Answer from the drawing. Dimensions are ordinates in mm from the lowest x, y and z of the part. A direction names the side the tool comes from. Give positions to 0.01 mm unless a question says otherwise; leave off trailing zeros. Write each loop counter-clockwise with the first axis right and the second up, starting at its lowest first coordinate (ties: lowest second). Pieces come first, ordered by that corner, then holes. Notation, with made-up numbers: (28.5, 76) -> (39.5, 76) arc R17 cw to (39.5, 99) -> close; hole circle Ø8 at (36.5, 1). An arc over 180 degrees is marked (long way). Write item = value, one per line.
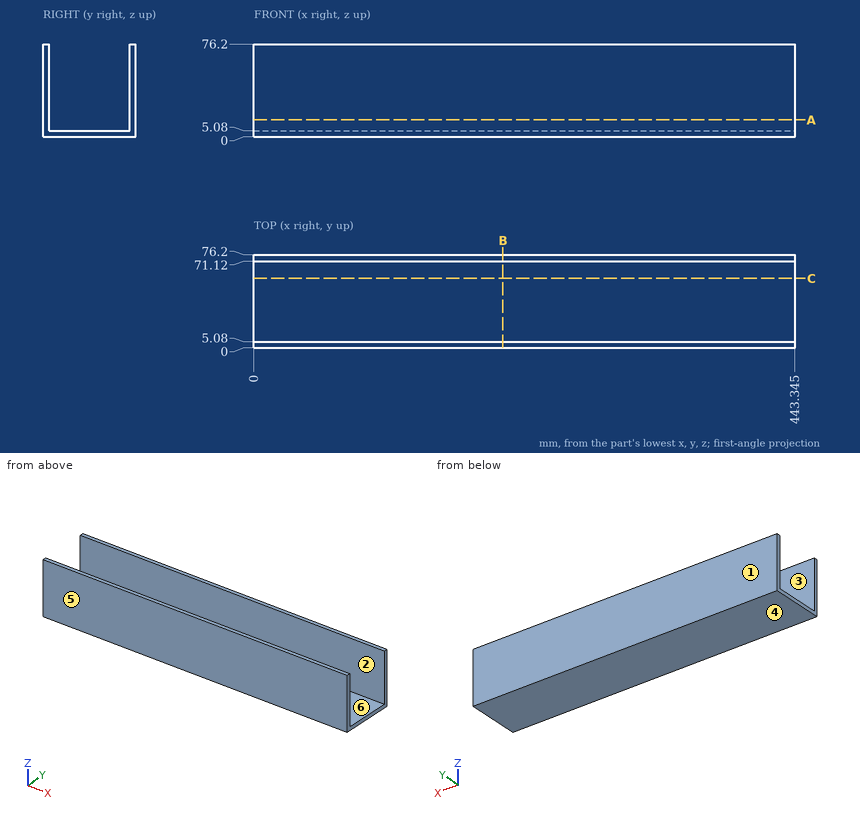
(1) For a pull along Y with two mould halves and no side action, classify the marked faces 3, 4, 5 and 6 as released by +Y, released by -Y, zero draft, split by the parting line, or undercut.
Checks:
face_3 = undercut
face_4 = zero draft
face_5 = released by -Y
face_6 = undercut
(2) Given P1, Ø5, axis at x = 126.5, y = 13, coming from the +Z side; P2, Ø8, axis at x = 189.5, y = 59, coming from the -Z side, each flat-ended and moving along its own axis, determine where each tip first touches the part or whether it passes through.
Checks:
P1 = 5.08
P2 = 0
(3) The part is cut by section B-B on x = 204. Determine the outline of the cut face in (y, z).
Checks:
outline = (0, 0) -> (76.2, 0) -> (76.2, 76.2) -> (71.12, 76.2) -> (71.12, 5.08) -> (5.08, 5.08) -> (5.08, 76.2) -> (0, 76.2) -> close
(4) A tool of negligible diameter and unlimited length cuts with its end or side. For the marked faces 1 and 2, from which of +Z, -Z, +X, -X, +Y, -Y can it reach the whole face along a straight path? Write none if from no direction.
Checks:
face_1 = +Z, -Z, +X, -X, +Y
face_2 = +Z, +X, -X
(5) Consider L1, parallel to Y at x = 384, z = 18; L2, parallel to Z at x = 186, y = 21. Determine where each line is inside the solid, lowest interval first.
Checks:
L1 = 0 to 5.08, 71.12 to 76.2
L2 = 0 to 5.08
(6) The part is cut by section C-C on y = 57. Determine the outline of the cut face in (x, z) (1 decimal), plus the area to 3 significant figures.
Checks:
outline = (0, 0) -> (443.3, 0) -> (443.3, 5.1) -> (0, 5.1) -> close
area = 2,250 mm²
(7) The part is cut by section A-A on z = 14. Determine the outline of the cut face in (x, y) (1 decimal).
Checks:
outline = (0, 0) -> (443.3, 0) -> (443.3, 5.1) -> (0, 5.1) -> close; (0, 71.1) -> (443.3, 71.1) -> (443.3, 76.2) -> (0, 76.2) -> close
